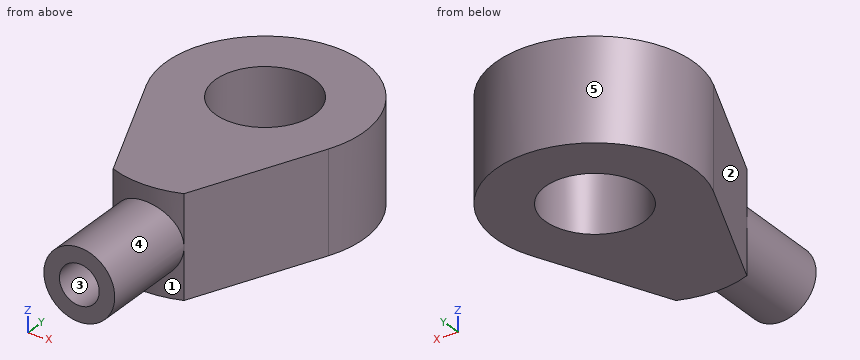
```python
from build123d import *

# Parameters (mm, degrees)
SKETCH1_R           = 2.5
BOSS_EXTRUDE1_DEPTH = 2.5535
SKETCH2_W           = 0.783
SKETCH2_H           = 5


with BuildPart() as part:
    # Sketch1 → Boss-Extrude1 (new, symmetric)
    with BuildSketch(Plane.XY):
        with BuildLine():
            Line((-4.582575695, -2), (-1.782575695, -8.415605973))
            ThreePointArc((-1.782575695, -8.415605973), (0, -8.744158243), (1.782575695, -8.415605973))
            Line((1.782575695, -8.415605973), (4.582575695, -2))
            ThreePointArc((4.582575695, -2), (0, 5), (-4.582575695, -2))
        make_face()
        with Locations(Location((0, 0, 0), (0, 0, 180))):
            Circle(SKETCH1_R, mode=Mode.SUBTRACT)
    extrude(amount=BOSS_EXTRUDE1_DEPTH, both=True)

    # Sketch2 → Revolve1 (revolve)
    with BuildSketch(Plane.XY, mode=Mode.PRIVATE) as revolve1_sk:
        with Locations((1.3915, -10.916)):
            Rectangle(SKETCH2_W, SKETCH2_H)
    revolve(revolve1_sk.sketch.rotate(Axis((0, -8.744158243, 0), (0, -1, 0)), 180), axis=Axis((0, -8.744158243, 0), (0, -1, 0)))


solid = part.part
```
The listing builds one solid part. Answer for the finished solid, in the listing's coordinates (mm). Face numbers are marked on the shaded views. A direction names the side the tool comes from. Give positions to 0.01 mm unless a question says otherwise; leave off trailing zeros. Order: outer loops, then holes, each group sorted by start corner. A loop starts at its lowest first (then second) coordinate and runs counter-clockwise, first axis right, second up. Notation, with made-up numbers: (47.25, 27.25) - (101.25, 27.25) arc R33 ccw to (101.25, 59.25) - close; hole circle Ø3 at (66.25, 18). An arc over 180 degrees is marked (long way). Use one line per item in the form item = value. Start each with the question number.
(1) Consider line 1 (Z direction, x = 0, y = -12); line 2 (Y direction, x = 1.75, z = 1.75); line 3 (Y direction, x = -2, z = 1.65). Determine where each line is inside the solid, lowest interval first. Write a range as from..to.
(2) A cutting plane is placed at D-D, the plane z = -0.4. Write down the section's boundary in (x, y).
(3) A cutting plane is placed at A-A, the plane y = 0. Write down the section's boundary in (x, z).
(4) The mould has two halves that part along Z. Classify the marked faces 3, 4 and 5: released by +Z, released by -Z, zero draft, split by the parting line, or undercut.
(5) A cutting plane is placed at C-C, the plane z = 0.5. Write down the section's boundary in (x, y), then the cut area to 3 significant figures.
(6) A cutting plane is placed at B-B, the plane x = 0. Write down the section's boundary in (y, z).
(7) For the marked faces 1 and 2, determine the directions among +Z, -Z, +X, -X, +Y, -Y from which every point of the face is accessible in a straight line to the end or side of a thin tool.
Ans:
q1.line_1 = -1.78..-1, 1..1.78
q1.line_2 = -8.43..-1.79, 1.79..4.68
q1.line_3 = -7.92..-1.5, 1.5..4.58
q2.outline = (-4.58, -2) - (-1.78, -8.42) arc R5 ccw to (-1.74, -8.43) - (-1.74, -13.42) - (-0.92, -13.42) - (-0.92, -8.66) arc R5 ccw to (0.92, -8.66) - (0.92, -13.42) - (1.74, -13.42) - (1.74, -8.43) arc R5 ccw to (1.78, -8.42) - (4.58, -2) arc R5 ccw (long way) to start; hole circle Ø5 at (0, 0)
q3.outline = (-5, -2.55) - (-2.5, -2.55) - (-2.5, 2.55) - (-5, 2.55) - close; (2.5, -2.55) - (5, -2.55) - (5, 2.55) - (2.5, 2.55) - close
q4.face_3 = undercut
q4.face_4 = split by the parting line
q4.face_5 = zero draft
q5.outline = (-4.58, -2) - (-1.78, -8.42) arc R5 ccw to (-1.71, -8.44) - (-1.71, -13.42) - (-0.87, -13.42) - (-0.87, -8.67) arc R5 ccw to (0.87, -8.67) - (0.87, -13.42) - (1.71, -13.42) - (1.71, -8.44) arc R5 ccw to (1.78, -8.42) - (4.58, -2) arc R5 ccw (long way) to start; hole circle Ø5 at (0, 0)
q5.area = 88.9 mm^2
q6.outline = (-13.42, -1.78) - (-8.74, -1.78) - (-8.74, -2.55) - (-2.5, -2.55) - (-2.5, 2.55) - (-8.74, 2.55) - (-8.74, 1.78) - (-13.42, 1.78) - (-13.42, 1) - (-8.74, 1) - (-8.74, -1) - (-13.42, -1) - close; (2.5, -2.55) - (5, -2.55) - (5, 2.55) - (2.5, 2.55) - close
q7.face_1 = -Y
q7.face_2 = +Z, -Z, -X, -Y
